Read the model definition and answer for the solid it produces. Units are mm, in the model's axes. A direction names the side the tool comes from. Coordinates: 2 decimals unless noted, no trailing zeros. Order: outer loops, then holes, each group sorted by start corner. A loop starts at its lowest first (then second) coordinate and runs counter-clockwise, first axis right, second up. Notation, with made-up numbers: M 24.25,71.5 L 29.25,71.5 A25 cw 29.25,96.5 Z; hole C -28.5,59.25 d10. An arc over 180 degrees is marked long. One line per question, with ' | ' between items. Start each with the question number.
1) Find section B-B, the plane x = 0. Write down the section's boundary in (y, z).
2) The mould has two halves that part along X. Classify faces 1 (the face through (-1, 0, 1)), 2 (the face through (0, 13.5, 0)), 3 (the face through (-2.75, 10.35, 62.44)): +X half, -X half, draft (parallel to the pull), parting line (faces both ways), or undercut.
3) Find section C-C, the plane z = 0. Write down the section's boundary in (x, y), plus the area to 3 significant figures.
4) Find section A-A, the plane y = 9. Write down the section's boundary in (x, z), plus the area to 3 significant figures.
5) A tool of negligible diameter and unlimited length cuts with its end or side. For faces 4 (the face through (13, 21, -27)), 5 (the face through (-26.36, 13.11, -5.85)), from which of +Z, -Z, +X, -X, +Y, -Y can it reach the whole face along a straight path? Write none if from no direction.
6) Find section D-D, the plane z = -16.5. Write down the section's boundary in (x, y), plus the area to 3 significant figures.
7) Consider probe 1 along X at (y, z) = (16, 0); probe 2 along X at (y, z) = (13.25, 0); probe 3 along Z at (x, y) = (-14.5, 18.25). Determine where each line is inside the solid, lowest interval first.
8) Given P1, Ø4, axis at x = -0.5, z = -0.5, coming from the +Y side; P2, Ø8, axis at x = -14, y = 2.5, coming from the +Z side; P3, Ø2, axis at y = 17, z = -22.5, coming from the +X side, each flat-ended and moving along its own axis, determine where each tip first touches the part or whether it passes through.
from build123d import *

# Parameters (mm, degrees)
SKETCH1_R           = 62.5
BOSS_EXTRUDE1_DEPTH = 21
SKETCH2_R           = 27
SKETCH2_R_2         = 6
CUT_EXTRUDE1_DEPTH  = 16
SKETCH3_R           = 6
SKETCH3_R_2         = 4
CUT_EXTRUDE2_DEPTH  = 14
SKETCH4_R           = 4
CUT_EXTRUDE3_DEPTH  = 7.5


with BuildPart() as part:
    # Sketch1 → Boss-Extrude1 (new body)
    with BuildSketch(Plane(origin=(0, 0, 0), x_dir=(1, 0, 0), z_dir=(0, 1, 0))):
        with Locations(Location((0, 0, 0), (0, 0, 90))):
            Circle(SKETCH1_R)
    extrude(amount=BOSS_EXTRUDE1_DEPTH)

    # Sketch2 → Cut-Extrude1 (cut)
    with BuildSketch(Plane(origin=(0, 21, 0), x_dir=(1, 0, 0), z_dir=(0, 1, 0))):
        with Locations(Location((0, 0, 0), (0, 0, 270))):
            Circle(SKETCH2_R)
        with Locations(Location((0, 0, 0), (0, 0, 270))):
            Circle(SKETCH2_R_2, mode=Mode.SUBTRACT)
    extrude(amount=-CUT_EXTRUDE1_DEPTH, mode=Mode.SUBTRACT)

    # Sketch3 → Cut-Extrude2 (cut)
    with BuildSketch(Plane(origin=(0, 21, 0), x_dir=(1, 0, 0), z_dir=(0, 1, 0))):
        with Locations(Location((0, 0, 0), (0, 0, 270))):
            Circle(SKETCH3_R)
        with Locations(Location((0, 0, 0), (0, 0, 270))):
            Circle(SKETCH3_R_2, mode=Mode.SUBTRACT)
    extrude(amount=-CUT_EXTRUDE2_DEPTH, mode=Mode.SUBTRACT)

    # Sketch4 → Cut-Extrude3 (cut)
    with BuildSketch(Plane(origin=(0, 21, 0), x_dir=(1, 0, 0), z_dir=(0, 1, 0))):
        with Locations(Location((0, 0, 0), (0, 0, 270))):
            Circle(SKETCH4_R)
    extrude(amount=-CUT_EXTRUDE3_DEPTH, mode=Mode.SUBTRACT)


solid = part.part
Report:
1) outline: M 0,-62.5 L 21,-62.5 L 21,-27 L 5,-27 L 5,-6 L 7,-6 L 7,-4 L 13.5,-4 L 13.5,4 L 7,4 L 7,6 L 5,6 L 5,27 L 21,27 L 21,62.5 L 0,62.5 Z
2) face 1: draft | face 2: undercut | face 3: parting line
3) outline: M -62.5,0 L 62.5,0 L 62.5,21 L 27,21 L 27,5 L 6,5 L 6,7 L 4,7 L 4,13.5 L -4,13.5 L -4,7 L -6,7 L -6,5 L -27,5 L -27,21 L -62.5,21 Z | area: 1,840 mm^2
4) outline: C 0,0 d125; C 0,0 d8; hole C 0,0 d54 | area: 10,000 mm^2
5) face 4: +Z, -Z, +X, -X, +Y | face 5: +Y
6) outline: M -60.28,0 L 60.28,0 L 60.28,21 L 21.37,21 L 21.37,5 L -21.37,5 L -21.37,21 L -60.28,21 Z | area: 1,850 mm^2
7) probe 1: x = -62.5 to -27, 27 to 62.5 | probe 2: x = -62.5 to -27, -4 to 4, 27 to 62.5 | probe 3: z = -60.79 to -22.78, 22.78 to 60.79
8) P1: stops at y = 13.5 | P2: stops at z = 61.69 | P3: stops at x = 58.69
